Could you check a few things on this drawing? It's one solid part, dimensions in mm from its lowest x, y, z. A direction names the side the tool comes from. Give positions to 0.01 mm unless a question says otherwise; leave off trailing zeros. Write each loop counter-clockwise with the first axis right and the second up, starting at its lowest first coordinate (ties: lowest second). Pieces come first, ordered by that corner, then holes. Notation, with made-up numbers: (-34.75, 8.5) - (-22.75, 8.5) arc R27 cw to (-22.75, 33.5) - close; hole circle Ø11 at (-27.75, 37.25). An arc over 180 degrees is marked (long way). One line per item, written item: value. Start each with the question number.
1) On a 3-axis mill with a long thin cutter (end or side, diameter ignored), from which of +Z, -Z, +X, -X, +Y, -Y can I reach the whole of each face in a straight line? I mean the marked faces 1 and 2. Say none if no direction works.
2) Please list where this line runs through material, in increasing order: L1, parallel to X at y = 8.5, z = 17.5. Write a range as [from, to].
3) I'm going to push flat-ended pins straight in: P1, Ø5, axis at x = 46.5, z = 11, coming from the +Y side; P2, Ø1.5, axis at y = 31, z = 33, coming from the +X side; P3, Ø3, axis at x = 19.5, y = 39, coming from the +Z side. Where does each tip first touch, or does it pass through?
4) Imagine slicing it at A-A on x = 15. Write out the boundary of the cut face in (y, z), plus the area to 3 significant figures.
5) Imagine slicing it at B-B on y = 49.5. Write out the boundary of the cut face in (x, z), plus the area to 3 significant figures.
6) Imagine slicing it at C-C on z = 23. Write out the boundary of the cut face in (x, y).
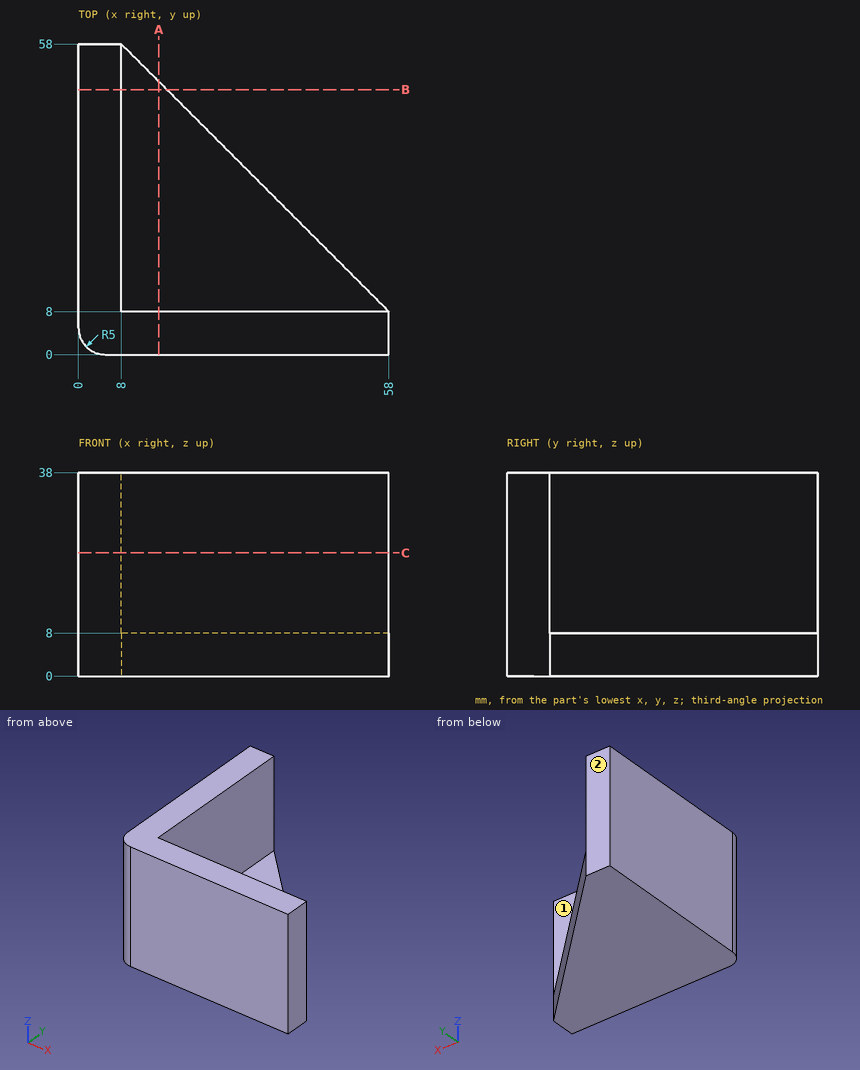
Numbers:
1. face 1: +Z, +X, +Y
1. face 2: +Z, -Z, +X, -X, +Y
2. L1: [0, 8]
3. P1: y = 8
3. P2: x = 8
3. P3: z = 8
4. outline: (0, 0) - (51, 0) - (51, 8) - (8, 8) - (8, 38) - (0, 38) - close
4. area: 648 mm^2
5. outline: (0, 0) - (16.5, 0) - (16.5, 8) - (8, 8) - (8, 38) - (0, 38) - close
5. area: 372 mm^2
6. outline: (0, 5) arc R5 ccw to (5, 0) - (58, 0) - (58, 8) - (8, 8) - (8, 58) - (0, 58) - close
